The model under review builds one solid part; all positions refer to its coordinate system, in mm. Coordinates: 2 decimals unless noted, no trailing zeros. Order: outer loops, then holes, each group sorted by start corner. A loop starts at its lowest first (then second) coordinate and runs counter-clockwise, first axis right, second up. Notation, with made-up numbers: M 78.5,80.5 L 126.5,80.5 A29 cw 126.5,106.5 Z; hole C -4,-31.75 d4. An arc over 180 degrees is marked long. Answer in a Markdown table with one row per item.
from build123d import *

# Parameters (mm, degrees)
SKETCH1_W           = 432
SKETCH1_H           = 200
BOSS_EXTRUDE1_DEPTH = 2.5
SKETCH3_R           = 7
SKETCH3_R_2         = 2
SKETCH3_W           = 498.20945101
SKETCH3_H           = 57.36356312
CUT_EXTRUDE1_DEPTH  = 2.5
SKETCH5_W           = 366.875294571
SKETCH5_H           = 10
SKETCH5_W_2         = 65.124705429
CUT_EXTRUDE3_DEPTH  = 2.5
SKETCH6_R           = 2
CUT_EXTRUDE4_DEPTH  = 2.5
CUT_EXTRUDE5_DEPTH  = 2.5
FILLET1_SIZE        = 30
SKETCH9_R           = 2
CUT_EXTRUDE6_DEPTH  = 2.5
SKETCH10_R          = 2
CUT_EXTRUDE7_DEPTH  = 2.5
SKETCH6_3_R         = 18.75
CUT_EXTRUDE8_DEPTH  = 10
SKETCH12_R          = 7
SKETCH12_R_2        = 2
CUT_EXTRUDE9_DEPTH  = 10


with BuildPart() as part:
    # Sketch1 → Boss-Extrude1 (new body)
    with BuildSketch(Plane(origin=(0, 0, 0), x_dir=(1, 0, 0), z_dir=(0, 1, 0))):
        with Locations((112.865968756, 71.914913526)):
            Rectangle(SKETCH1_W, SKETCH1_H)
    extrude(amount=BOSS_EXTRUDE1_DEPTH)

    # Sketch3 → Cut-Extrude1 (cut)
    with BuildSketch(Plane(origin=(0, 2.5, 0), x_dir=(1, 0, 0), z_dir=(0, 1, 0))):
        with Locations(Location((-13.134031244, 71.914913526, 0), (0, 0, 270))):
            Circle(SKETCH3_R)
        with Locations(Location((-29.135857702, 55.913087067, 0), (0, 0, 270))):
            Circle(SKETCH3_R_2)
        with Locations(Location((-29.135857702, 87.916739984, 0), (0, 0, 270))):
            Circle(SKETCH3_R_2)
        with Locations(Location((2.867795214, 55.913087067, 0), (0, 0, 270))):
            Circle(SKETCH3_R_2)
        with Locations(Location((2.867795214, 87.916739984, 0), (0, 0, 270))):
            Circle(SKETCH3_R_2)
        with Locations(Location((238.865968756, 71.914913526, 0), (0, 0, 270))):
            Circle(SKETCH3_R)
        with Locations((79.761243251, 144.596695086)):
            Rectangle(SKETCH3_W, SKETCH3_H)
        with Locations(Location((222.864142298, 55.913087067, 0), (0, 0, 270))):
            Circle(SKETCH3_R_2)
        with Locations(Location((254.867795214, 87.916739984, 0), (0, 0, 270))):
            Circle(SKETCH3_R_2)
        with Locations(Location((222.864142298, 87.916739984, 0), (0, 0, 270))):
            Circle(SKETCH3_R_2)
        with Locations(Location((254.867795214, 55.913087067, 0), (0, 0, 270))):
            Circle(SKETCH3_R_2)
    extrude(amount=-CUT_EXTRUDE1_DEPTH, mode=Mode.SUBTRACT)

    # Sketch5 → Cut-Extrude3 (cut)
    with BuildSketch(Plane(origin=(0, 2.5, 0), x_dir=(1, 0, 0), z_dir=(0, 1, 0))):
        with Locations((80.303616041, -23.085086474)):
            Rectangle(SKETCH5_W, SKETCH5_H)
        with Locations((296.303616042, -23.085086474)):
            Rectangle(SKETCH5_W_2, SKETCH5_H)
    extrude(amount=-CUT_EXTRUDE3_DEPTH, mode=Mode.SUBTRACT)

    # Sketch6 → Cut-Extrude4 (cut)
    with BuildSketch(Plane(origin=(0, 2.5, 0), x_dir=(1, 0, 0), z_dir=(0, 1, 0))):
        with Locations(Location((71.864142298, 5.913087067, 0), (0, 0, 270))):
            Circle(SKETCH6_R)
        with Locations(Location((71.864142298, 37.916739984, 0), (0, 0, 270))):
            Circle(SKETCH6_R)
        with Locations(Location((103.867795214, 37.916739984, 0), (0, 0, 270))):
            Circle(SKETCH6_R)
        with Locations(Location((103.867795214, 5.913087067, 0), (0, 0, 270))):
            Circle(SKETCH6_R)
        with Locations(Location((121.864142298, 5.913087067, 0), (0, 0, 270))):
            Circle(SKETCH6_R)
        with Locations(Location((121.864142298, 37.916739984, 0), (0, 0, 270))):
            Circle(SKETCH6_R)
        with Locations(Location((153.867795214, 37.916739984, 0), (0, 0, 270))):
            Circle(SKETCH6_R)
        with Locations(Location((153.867795214, 5.913087067, 0), (0, 0, 270))):
            Circle(SKETCH6_R)
    extrude(amount=-CUT_EXTRUDE4_DEPTH, mode=Mode.SUBTRACT)

    # Sketch8 → Cut-Extrude5 (cut)
    with BuildSketch(Plane(origin=(0, 2.5, 0), x_dir=(1, 0, 0), z_dir=(0, 1, 0))):
        with BuildLine():
            Line((176.582305496, -4.412929011), (152.923062834, 63.765083659))
            ThreePointArc((152.923062834, 63.765083659), (153.539952677, 65.037658577), (154.812527595, 64.420768733))
            Line((154.812527595, 64.420768733), (178.471770257, -3.757243937))
            ThreePointArc((178.471770257, -3.757243937), (177.854880414, -5.029818855), (176.582305496, -4.412929011))
        make_face()
        with BuildLine():
            Line((47.260167255, -3.757243937), (70.919409917, 64.420768733))
            ThreePointArc((70.919409917, 64.420768733), (72.191984835, 65.037658577), (72.808874679, 63.765083659))
            Line((72.808874679, 63.765083659), (49.149632016, -4.412929011))
            ThreePointArc((49.149632016, -4.412929011), (47.877057099, -5.029818855), (47.260167255, -3.757243937))
        make_face()
    extrude(amount=-CUT_EXTRUDE5_DEPTH, mode=Mode.SUBTRACT)

    # Fillet1
    # a fillet whose section is not a circle: 30 mm, written as the material it takes off along each edge
    with BuildSketch(Plane(origin=(-103.134031244, -75, -115.914913526), x_dir=(0, 0, 1), z_dir=(0, 1, 0)), Plane(origin=(-103.134031244, 77.5, 18.085086474), x_dir=(0, 0, -1), z_dir=(0, -1, 0)), Plane(origin=(328.865968756, 77.5, 18.085086474), x_dir=(-1, 0, 0), z_dir=(0, -1, 0))) as fillet1_piece_1:
        with BuildLine():
            add(Edge.make_bspline([(FILLET1_SIZE, 0), (FILLET1_SIZE * 0.831801948466, 0), (FILLET1_SIZE * 0.663603896932, 0), (FILLET1_SIZE * 0.292893218813, FILLET1_SIZE * 0.0716919198361), (FILLET1_SIZE * 0.0716919198361, FILLET1_SIZE * 0.292893218813), (0, FILLET1_SIZE * 0.663603896932), (0, FILLET1_SIZE * 0.831801948466), (0, FILLET1_SIZE)], knots=[0, 0, 0, 0, 0, 0, 0.5, 0.5, 1, 1, 1, 1, 1, 1], degree=5))
            Line((0, FILLET1_SIZE), (0, 0))
            Line((0, 0), (FILLET1_SIZE, 0))
        make_face()
    extrude(amount=152.5, mode=Mode.SUBTRACT)
    with BuildSketch(Plane(origin=(328.865968756, 77.5, -115.914913526), x_dir=(-1, 0, 0), z_dir=(0, -1, 0))) as fillet1_piece_2:
        with BuildLine():
            add(Edge.make_bspline([(FILLET1_SIZE, 0), (FILLET1_SIZE * 0.831801948466, 0), (FILLET1_SIZE * 0.663603896932, 0), (FILLET1_SIZE * 0.292893218813, -FILLET1_SIZE * 0.0716919198361), (FILLET1_SIZE * 0.0716919198361, -FILLET1_SIZE * 0.292893218813), (0, -FILLET1_SIZE * 0.663603896932), (0, -FILLET1_SIZE * 0.831801948466), (0, -FILLET1_SIZE)], knots=[0, 0, 0, 0, 0, 0, 0.5, 0.5, 1, 1, 1, 1, 1, 1], degree=5))
            Line((0, -FILLET1_SIZE), (0, 0))
            Line((0, 0), (FILLET1_SIZE, 0))
        make_face()
    extrude(amount=152.5, mode=Mode.SUBTRACT)

    # Sketch9 → Cut-Extrude6 (cut)
    with BuildSketch(Plane(origin=(0, 2.5, 0), x_dir=(1, 0, 0), z_dir=(0, 1, 0))):
        with Locations(Location((321.865968752, 6.010283068, 0), (0, 0, 270))):
            Circle(SKETCH9_R)
        with Locations(Location((321.865968752, 48.914945481, 0), (0, 0, 270))):
            Circle(SKETCH9_R)
        with Locations(Location((321.865968752, 91.819607898, 0), (0, 0, 270))):
            Circle(SKETCH9_R)
        with Locations(Location((-96.134031244, 46.467317494, 0), (0, 0, 270))):
            Circle(SKETCH9_R)
        with Locations(Location((-96.134031244, 91.819607898, 0), (0, 0, 270))):
            Circle(SKETCH9_R)
        with Locations(Location((-96.134031244, 6.010283068, 0), (0, 0, 270))):
            Circle(SKETCH9_R)
    extrude(amount=-CUT_EXTRUDE6_DEPTH, mode=Mode.SUBTRACT)

    # Sketch10 → Cut-Extrude7 (cut)
    with BuildSketch(Plane(origin=(0, 2.5, 0), x_dir=(1, 0, 0), z_dir=(0, 1, 0))):
        with Locations(Location((112.866022655, -8.085086472, 0), (0, 0, 270))):
            Circle(SKETCH10_R)
        with Locations(Location((294.941757967, -8.085086472, 0), (0, 0, 270))):
            Circle(SKETCH10_R)
        with Locations(Location((-69.209712656, -8.085086472, 0), (0, 0, 270))):
            Circle(SKETCH10_R)
    extrude(amount=-CUT_EXTRUDE7_DEPTH, mode=Mode.SUBTRACT)

    # Sketch6<3> → Cut-Extrude8 (cut)
    with BuildSketch(Plane(origin=(0, 2.5, 0), x_dir=(1, 0, 0), z_dir=(0, 1, 0))):
        with Locations(Location((137.865968756, 21.914913526, 0), (0, 0, 270))):
            Circle(SKETCH6_3_R)
        with Locations(Location((87.865968756, 21.914913526, 0), (0, 0, 270))):
            Circle(SKETCH6_3_R)
    extrude(amount=-CUT_EXTRUDE8_DEPTH, mode=Mode.SUBTRACT)

    # Sketch12 → Cut-Extrude9 (cut)
    with BuildSketch(Plane(origin=(0, 2.5, 0), x_dir=(1, 0, 0), z_dir=(0, 1, 0))):
        with Locations(Location((121.864142298, 71.914913526, 0), (0, 0, 270))):
            Circle(SKETCH12_R)
        with Locations(Location((105.86231584, 55.913087067, 0), (0, 0, 270))):
            Circle(SKETCH12_R_2)
        with Locations(Location((105.86231584, 87.916739984, 0), (0, 0, 270))):
            Circle(SKETCH12_R_2)
        with Locations(Location((137.865968756, 87.916739984, 0), (0, 0, 270))):
            Circle(SKETCH12_R_2)
        with Locations(Location((137.865968756, 55.913087067, 0), (0, 0, 270))):
            Circle(SKETCH12_R_2)
    extrude(amount=-CUT_EXTRUDE9_DEPTH, mode=Mode.SUBTRACT)


solid = part.part
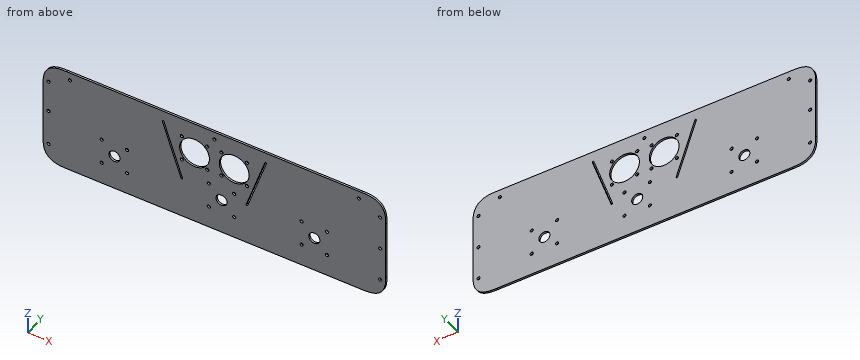
(1) Take a section at A-A (x = 93.5). Write out the cut boundary in (y, z), then the cut area to 3 significant figures.
Report:
| item | result |
|---|---|
| outline | M 0,-115.91 L 2.5,-115.91 L 2.5,-39.8 L 0,-39.8 Z; M 0,-4.03 L 2.5,-4.03 L 2.5,18.09 L 0,18.09 Z |
| area | 246 mm^2 |
(2) To check wall thickness, follow line 1 (X direction, y = 0.25, z = 0); line 2 (X direction, y = 1.15, z = -61); line 3 (X direction, y = 2.25, z = -22.5). State the ranges of each line that lie inside material, in increasing order. Write a range as [from, to].
Report:
| item | result |
|---|---|
| line 1 | [-102.25, 48.56], [50.68, 175.05], [177.17, 327.99] |
| line 2 | [-103.13, 69.73], [71.85, 153.88], [156, 328.87] |
| line 3 | [-103.13, 56.37], [58.49, 69.13], [106.61, 119.13], [156.61, 167.24], [169.36, 328.87] |
(3) Insertion check: P1, Ø3, axis at x = 294.94, z = 8.09, coming from the -Y side. The pin has a flat end and moves straight along its axis. Give the tip position at first contact, or say it passes through.
Report:
| item | result |
|---|---|
| P1 | through |
(4) Take a section at B-B (z = -69.5). Write out the cut boundary in (x, y).
Report:
| item | result |
|---|---|
| outline | M -103.13,0 L -19.7,0 L -19.7,2.5 L -103.13,2.5 Z; M -6.56,0 L 115.29,0 L 115.29,2.5 L -6.56,2.5 Z; M 128.43,0 L 232.3,0 L 232.3,2.5 L 128.43,2.5 Z; M 245.44,0 L 328.87,0 L 328.87,2.5 L 245.44,2.5 Z |
(5) Take a section at C-C (y = 0.55). State how many separate pieces and enclosed holes the cut face has, then the cut area to 3 significant figures.
Report:
| item | result |
|---|---|
| separate pieces | 1 |
| enclosed holes | 36 |
| area | 54,100 mm^2 |
